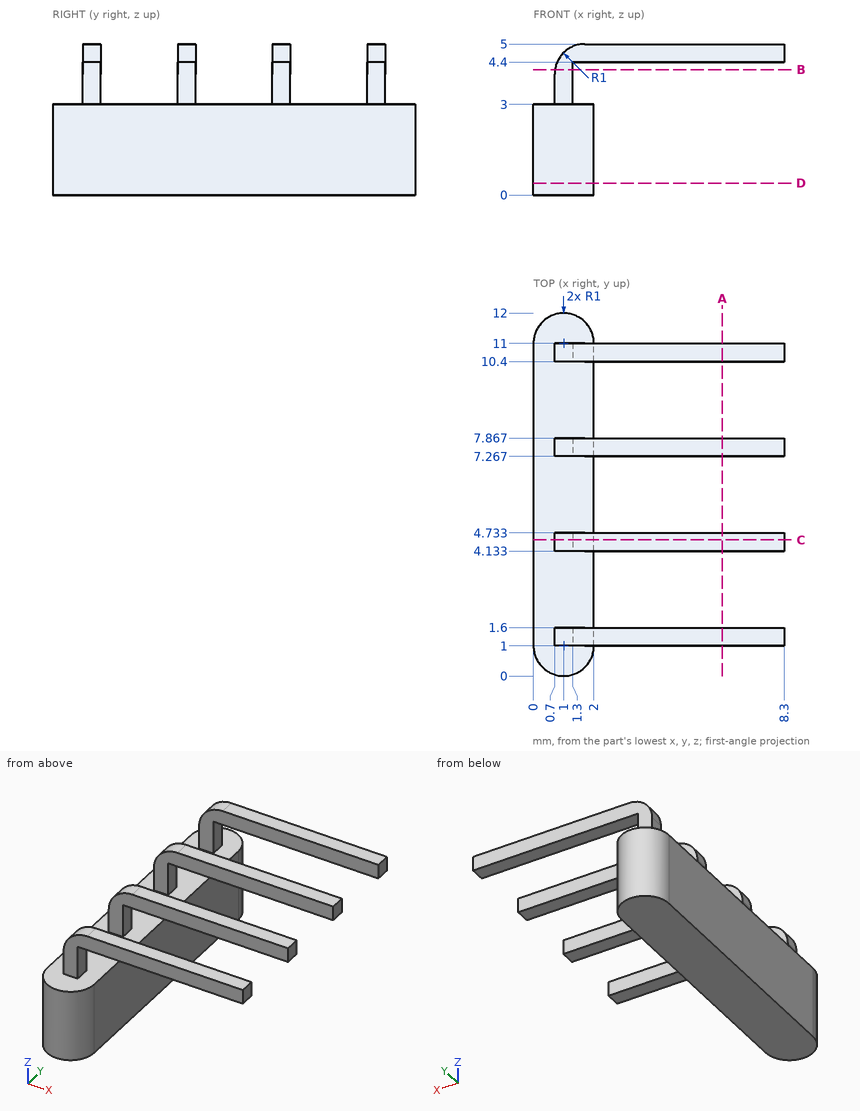
Input: dimensioned drawing with shaded views. Units: mm. Origin: part minimum x, y, z. Round coordinates to 2 decimals unless told otherwise and drop trailing zeros. Loops run counter-clockwise (first coordinate to the right, second up) from the corner with the lowest first, then second, coordinate; pieces in that order, holes last. Notation, with made-up numbers: M 20,9.5 L 36,9.5 A12 cw 36,13.5 Z; hole C -4.75,65 d10. An arc over 180 degrees is marked long. Return JSON: item names as keys, results as strings. Group by question number.
1. Pin query (flat end, axial travel): pin 1 (0.5 mm diameter, centred on y = 4.5, z = 4, fed in from +X); pin 2 (0.5 mm diameter, centred on y = 1.5, z = 3.5, fed in from -X); pin 3 (3 mm diameter, centred on x = 6, z = 4, fed in from -Y); pin 4 (1 mm diameter, centred on y = 5.5, z = 1, fed in from -X). Return the tip coordinate at first contact, or that it passes through.
2. Section query B-B on z = 4.15. Output: boundary loops of the cut face in (x, y).
3. Section query C-C on y = 4.5. Output: boundary loops of the cut face in (x, z).
4. Section query A-A on x = 6.25. Output: boundary loops of the cut face in (y, z).
5. Material intervals for line 1 along Y through (x, z) = (3, 4.75); line 2 along X through (y, z) = (5.5, 1.25); line 3 along Z through (x, y) = (1.5, 6), sorted ascending. Write a range as from..to.
6. Section query D-D on z = 0.4. Output: boundary loops of the cut face in (x, y).
Checks:
{
 "1": {"pin 1": "stops at x = 1.3", "pin 2": "stops at x = 0.7", "pin 3": "stops at y = 1", "pin 4": "stops at x = 0"},
 "2": {"outline": "M 0.71,1 L 1.3,1 L 1.3,1.6 L 0.71,1.6 Z; M 0.71,4.13 L 1.3,4.13 L 1.3,4.73 L 0.71,4.73 Z; M 0.71,7.27 L 1.3,7.27 L 1.3,7.87 L 0.71,7.87 Z; M 0.71,10.4 L 1.3,10.4 L 1.3,11 L 0.71,11 Z"},
 "3": {"outline": "M 0,0 L 2,0 L 2,3 L 1.3,3 L 1.3,4.4 L 8.3,4.4 L 8.3,5 L 1.7,5 A1 ccw 0.7,4 L 0.7,3 L 0,3 Z"},
 "4": {"outline": "M 1,4.4 L 1.6,4.4 L 1.6,5 L 1,5 Z; M 4.13,4.4 L 4.73,4.4 L 4.73,5 L 4.13,5 Z; M 7.27,4.4 L 7.87,4.4 L 7.87,5 L 7.27,5 Z; M 10.4,4.4 L 11,4.4 L 11,5 L 10.4,5 Z"},
 "5": {"line 1": "y = 1..1.6, 4.13..4.73, 7.27..7.87, 10.4..11", "line 2": "x = 0..2", "line 3": "z = 0..3"},
 "6": {"outline": "M 0,1 A1 ccw 2,1 L 2,11 A1 ccw 0,11 Z"}
}
